Work out the finished part from the listing and answer in its coordinate system (mm). Face numbers are marked on the shaded views. A direction names the side the tool comes from. Round coordinates to 2 decimals unless told otherwise and drop trailing zeros. Write each loop counter-clockwise with the first axis right and the second up, starting at its lowest first coordinate (ties: lowest second). Pieces come first, ordered by that corner, then holes.
1. Find section D-D (z = 8.5). Write down the section's boundary in (x, y).
2. Straight lines are drawn through the part: probe 1 along Z at (x, y) = (2.5, 0); probe 2 along X at (y, z) = (-2.5, 5.5); probe 3 along X at (y, z) = (1.5, 7). For each, find the intervals that lie inside material, in ascending order.
3. Find section B-B (y = -0.5). Write down the section's boundary in (x, z).
4. Determine the mould class of the marked faces 1, 2 and 3 for opening direction X: pulls with the +X half, pulls with the -X half, needs draft (parallel to the pull), parting line crosses it, or undercut.
5. Find section C-C (x = 5). Write down the section's boundary in (y, z).
6. Flat-ended cylindrical pins translate along their axes: pin 1 Ø4 at (x, y) = (-1.5, -3.5) entering from -Z; pin 2 Ø1.5 at (y, z) = (0.5, 8) entering from -X; pin 3 Ø1.5 at (x, y) = (-1, 0) entering from +Z; pin 4 Ø2 at (x, z) = (-17.5, 5.5) entering from -Y. Find the tip coordinate at first contact, or state that the pin passes through.
7. Find section A-A (z = 6.25). Write down the section's boundary in (x, y), and give its area (3 significant figures).
8. A tool of negligible diameter and unlimited length cuts with its end or side. For the marked faces 4 and 5, from which of +Z, -Z, +X, -X, +Y, -Y can it reach the whole face along a straight path? Write none if from no direction.
```python
from build123d import *

# Parameters (mm, degrees)
SKETCH1_W           = 10
SKETCH1_H           = 60
BOSS_EXTRUDE1_DEPTH = 10
DRAFT1_ANGLE        = -10
SKETCH2_W           = 5.08
SKETCH2_H           = 30
CUT_EXTRUDE1_DEPTH  = 5


with BuildPart() as part:
    # Sketch1 → Boss-Extrude1 (new body)
    with BuildSketch(Plane(origin=(0, 0, 0), x_dir=(0, 1, 0), z_dir=(0, 0, 1))):
        Rectangle(SKETCH1_W, SKETCH1_H)
    extrude(amount=BOSS_EXTRUDE1_DEPTH)

    # Draft1
    draft1_faces = [part.faces().sort_by_distance(p)[0] for p in [
        (-30, 0, 5),
        (0, -5, 5),
        (0, 5, 5),
        (30, 0, 5),
    ]]
    draft(draft1_faces, Plane(origin=(0, 0, 0), x_dir=(-1, 0, 0), z_dir=(0, 0, -1)), DRAFT1_ANGLE)

    # Sketch2 → Cut-Extrude1 (cut)
    with BuildSketch(Plane.XY.offset(10)):
        Rectangle(SKETCH2_W, SKETCH2_H)
    extrude(amount=-CUT_EXTRUDE1_DEPTH, mode=Mode.SUBTRACT)


solid = part.part
```
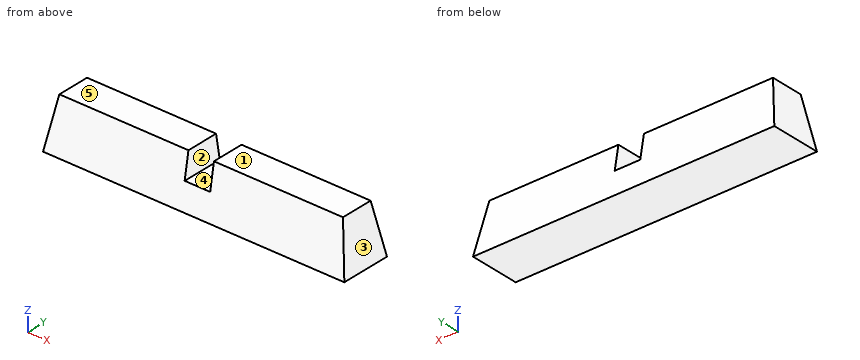
Worked answers:
1. outline: (-28.5, -3.5) - (-2.54, -3.5) - (-2.54, 3.5) - (-28.5, 3.5) - close; (2.54, -3.5) - (28.5, -3.5) - (28.5, 3.5) - (2.54, 3.5) - close
2. probe 1: z = 0 to 5
2. probe 2: x = -29.03 to -2.54, 2.54 to 29.03
2. probe 3: x = -28.77 to -2.54, 2.54 to 28.77
3. outline: (-30, 0) - (30, 0) - (28.24, 10) - (2.54, 10) - (2.54, 5) - (-2.54, 5) - (-2.54, 10) - (-28.24, 10) - close
4. face 1: needs draft
4. face 2: undercut
4. face 3: pulls with the +X half
5. outline: (-5, 0) - (5, 0) - (3.24, 10) - (-3.24, 10) - close
6. pin 1: stops at z = 0
6. pin 2: stops at x = -28.72
6. pin 3: stops at z = 5
6. pin 4: stops at y = -4.21
7. outline: (-28.9, -3.9) - (-2.54, -3.9) - (-2.54, 3.9) - (-28.9, 3.9) - close; (2.54, -3.9) - (28.9, -3.9) - (28.9, 3.9) - (2.54, 3.9) - close
7. area: 411 mm2
8. face 4: +Z, +Y, -Y
8. face 5: +Z, +X, -X, +Y, -Y
